Build history of the part. All positions in model axes, mm. Round coordinates to 2 decimals unless told otherwise and drop trailing zeros. Write each loop counter-clockwise with the first axis right and the second up, starting at its lowest first coordinate (ties: lowest second). Pieces come first, ordered by that corner, then holes. Notation, with made-up numbers: (33, 4) -> (91, 4) arc R16 cw to (91, 22) -> close; hole circle Ø7 at (-35.5, -9.75). An arc over 180 degrees is marked (long way). Return JSON: item names as keys, results as strings.
from build123d import *

# Parameters (mm, degrees)
SKETCH_1_W                   = 14
SKETCH_1_H                   = 6
EXTRUDE_1_DEPTH              = 2
HOLE_WIZARD_4_401_AT_2_COUNT = 2
HOLE_WIZARD_4_401_AT_2_PITCH = 8
CHAMFER_1_SIZE               = 1
CHAMFER_1_SIZE_2             = 1.428148007


with BuildPart() as part:
    # Эскиз1 → Бобышка-Вытянуть1 (new body)
    with BuildSketch(Plane(origin=(0, 0, 0), x_dir=(0, 0, -1), z_dir=(1, 0, 0))):
        Rectangle(SKETCH_1_W, SKETCH_1_H)
    extrude(amount=EXTRUDE_1_DEPTH)

    # Эскиз4 → Отверстие обработанное метчиком #4-401 (revolve, cut)
    with BuildSketch(Plane(origin=(2, 0, 4), x_dir=(0, 0, -1), z_dir=(0, 1, 0))):
        Polygon((0, 0), (0, 2), (1.778, 2), (1.4224, 1.751006199), (1.4224, 0.248993801), (1.778, 0), align=None)
    hole_wizard_4_401 = revolve(axis=Axis((8.35, 0, 4), (-1, 0, 0)), mode=Mode.SUBTRACT)

    # Отверстие обработанное метчиком #4-401 at 2: Отверстие обработанное метчиком #4-401 ×2
    with Locations(*[(0, 0, -i * HOLE_WIZARD_4_401_AT_2_PITCH) for i in range(1, HOLE_WIZARD_4_401_AT_2_COUNT)]):
        add(hole_wizard_4_401, mode=Mode.SUBTRACT)

    # Фаска1
    # the kernel refuses this chamfer: 1.428148007, 1 mm, written as the material it takes off along each edge
    with BuildSketch(Plane(origin=(0, 6.68826682, 7), x_dir=(0.9989750717851554, 0, 0.04526373771402103), z_dir=(0, -1, 0))) as chamfer_1_piece_1:
        Polygon((CHAMFER_1_SIZE * 0.998975071785, -CHAMFER_1_SIZE * 0.045263737714), (-CHAMFER_1_SIZE_2 * 0.0452637377058, -CHAMFER_1_SIZE_2 * 0.998975071605), (0, 0), align=None)
    extrude(amount=13.37653364, mode=Mode.SUBTRACT)


solid = part.part
Q1. Saw through at C-C on x = 1.25. List the corners of the cut face in (y, z), then the cut area to 3 significant figures.
Verdict:
{"outline": "(-3, -7) -> (3, -7) -> (3, 7) -> (-3, 7) -> close; hole circle Ø2.84 at (0, -4); hole circle Ø2.84 at (0, 4)", "area": "71.3 mm²"}
Q2. Saw through at A-A on z = 4. List the corners of the cut face in (x, y), then the cut area to 3 significant figures.
Verdict:
{"outline": "(0, -3) -> (2, -3) -> (2, -1.78) -> (1.75, -1.42) -> (0.25, -1.42) -> (0, -1.78) -> close; (0, 1.78) -> (0.25, 1.42) -> (1.75, 1.42) -> (2, 1.78) -> (2, 3) -> (0, 3) -> close", "area": "6.13 mm²"}
Q3. Wall check: L1, parallel to Z at x = 1.45, y = 0; L2, parallel to Y at x = 0.85, z = 4; L3, parallel to Z at x = 0.8, y = 0. Give the ranges that are in metal, low to high.
Verdict:
{"L1": "z = -7 to -5.42, -2.58 to 2.58, 5.42 to 7", "L2": "y = -3 to -1.42, 1.42 to 3", "L3": "z = -7 to -5.42, -2.58 to 2.58, 5.42 to 6.71"}
Q4. Saw through at D-D on y = 2.45. List the corners of the cut face in (x, z), then the cut area to 3 significant figures.
Verdict:
{"outline": "(0, -7) -> (2, -7) -> (2, 7) -> (1, 7) -> (0, 5.57) -> close", "area": "27.3 mm²"}
Q5. Two-plate mould, pull along Y, no slides. Class faces 1 (the cylindrical face through (1.011, 0.545, 2.686)), 2 (the flat face through (1, -3, 0)), 3 (the cylindrical face through (1.011, -0.427, -5.357)), 4 (the flat face through (1, 0, -7)): +Y half, -Y half, draft (parallel to the pull), parting line (faces both ways), or undercut.
Verdict:
{"face 1": "undercut", "face 2": "-Y half", "face 3": "undercut", "face 4": "draft"}
Q6. Pin check, flat tip, straight feed: pin 1 Ø3.5 at (y, z) = (0, -4) entering from +X. Stop position of the tip, or through.
Verdict:
{"pin 1": "stops at x = 1.98"}
Q7. Saw through at B-B on y = 0. List the corners of the cut face in (x, z), then the cut area to 3 significant figures.
Verdict:
{"outline": "(0, -7) -> (2, -7) -> (2, -5.78) -> (1.75, -5.42) -> (0.25, -5.42) -> (0, -5.78) -> close; (0, -2.22) -> (0.25, -2.58) -> (1.75, -2.58) -> (2, -2.22) -> (2, 2.22) -> (1.75, 2.58) -> (0.25, 2.58) -> (0, 2.22) -> close; (0.07, 5.67) -> (0.25, 5.42) -> (1.75, 5.42) -> (2, 5.78) -> (2, 7) -> (1, 7) -> close", "area": "15.6 mm²"}
